CAD build for the part. Positions are in the model's coordinates, mm. Face numbers are marked on the shaded views. A direction names the side the tool comes from. Give positions to 0.01 mm unless a question says otherwise; leave off trailing zeros. Loops run counter-clockwise (first coordinate to the right, second up) from the corner with the lowest first, then second, coordinate; pieces in that order, holes last.
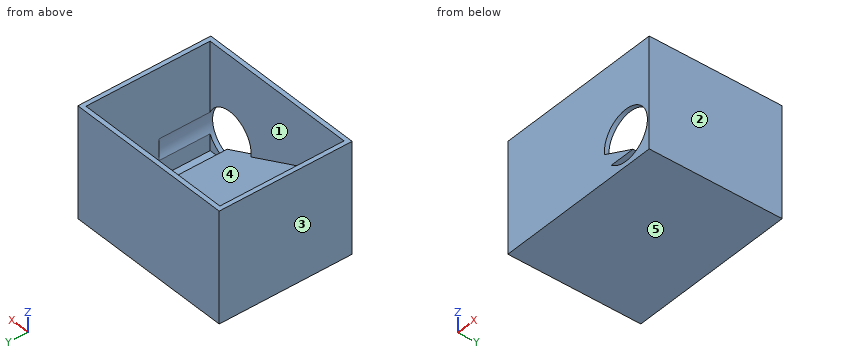
```python
from build123d import *

# Parameters (mm, degrees)
F0_W     = 76
F0_H     = 50
F1_DEPTH = 60
F2_W     = 72
F2_H     = 56
F3_DEPTH = 48.5
F4_R     = 11.544543
F5_DEPTH = 25
F7_DEPTH = 58


with BuildPart() as f1:
    # F0 (on Front) → F1 (new body)
    with BuildSketch(Plane.XZ):
        with Locations((1.184214, -10.245586)):
            Rectangle(F0_W, F0_H)
    extrude(amount=-F1_DEPTH)

    # F2 (on face) → F3 (cut)
    with BuildSketch(Plane.XY.offset(14.754414)):
        with Locations((1.184214, 30)):
            Rectangle(F2_W, F2_H)
    extrude(amount=-F3_DEPTH, mode=Mode.SUBTRACT)

    # F4 (on face) → F5 (cut)
    with BuildSketch(Plane.XZ):
        with Locations((26.681723, -21.490686)):
            Circle(F4_R)
    extrude(amount=-F5_DEPTH, mode=Mode.SUBTRACT)

    # F6 (on Front) → F7 (join)
    with BuildSketch(Plane.XZ):
        Polygon((-35.402854, 0), (-35.402854, -30), (30.412122, -30), align=None)
    extrude(amount=-F7_DEPTH)


solid = f1.part
```
1. Saw through at C-C, the plane z = 5.5. List the corners of the cut face in (x, y).
Responses:
outline: (-36.82, 0) - (39.18, 0) - (39.18, 60) - (-36.82, 60) - close; hole (-34.82, 2) - (37.18, 2) - (37.18, 58) - (-34.82, 58) - close
2. Probe line 1 along X through (y, z) = (56, 6); line 2 along Y through (x, z) = (-14, 12.5); line 3 along Y through (x, z) = (34.5, -19.5). List the from-to ranges inside material, lowest first.
Responses:
line 1: x = -36.82 to -34.82, 37.18 to 39.18
line 2: y = 0 to 2, 58 to 60
line 3: y = 58 to 60
3. Pull direction X, two halves, no side cores. Call the marked faces 3, 4 and 5: released by +X, released by -X, zero draft, split by the parting line, or undercut.
Responses:
face 3: released by -X
face 4: undercut
face 5: zero draft
4. Saw through at D-D, the plane x = 25. List the corners of the cut face in (y, z), and give its area (3 significant figures).
Responses:
outline: (0, -35.25) - (60, -35.25) - (60, 14.75) - (58, 14.75) - (58, -27.53) - (0, -27.53) - (0, -30) - (58, -30) - (58, -33.75) - (2, -33.75) - (2, -32.91) - (0, -32.91) - close; (0, -10.07) - (2, -10.07) - (2, 14.75) - (0, 14.75) - close
area: 381 mm2
5. Drop flat-ended pins along their axis: pin 1 (4 mm diameter, centred on x = 1, y = 40, fed in from +Z); pin 2 (2 mm diameter, centred on x = 9, y = 40, fed in from +Z). Give the stop position or say it passes through.
Responses:
pin 1: stops at z = -15.68
pin 2: stops at z = -19.78
6. Tool access for the marked faces 1 and 2: list every direction of +Z, -Z, +X, -X, +Y, -Y with a clear straight run to the whole face (end or side of a thin tool).
Responses:
face 1: +Z
face 2: +Z, -Z, +X, +Y, -Y
7. Saw through at A-A, the plane x = 16.5. List the corners of the cut face in (y, z), and give its area (3 significant figures).
Responses:
outline: (0, -35.25) - (60, -35.25) - (60, 14.75) - (58, 14.75) - (58, -23.66) - (0, -23.66) - close; (0, -16.05) - (2, -16.05) - (2, 14.75) - (0, 14.75) - close; hole (2, -33.75) - (58, -33.75) - (58, -30) - (2, -30) - close
area: 624 mm2
8. Saw through at B-B, the plane y = 5. List the corners of the cut face in (x, z).
Responses:
outline: (-36.82, -35.25) - (39.18, -35.25) - (39.18, 14.75) - (37.18, 14.75) - (37.18, -16.7) arc R11.54 cw to (37.18, -26.28) - (37.18, -33.75) - (-34.82, -33.75) - (-34.82, -30) - (30.41, -30) - (-34.82, -0.27) - (-34.82, 14.75) - (-36.82, 14.75) - close
